```python
from build123d import *

# Parameters (mm, degrees)
SKETCH1_W           = 26
SKETCH1_H           = 26
BOSS_EXTRUDE1_DEPTH = 155
SHELL1_T            = -3
SKETCH2_W           = 10
SKETCH2_H           = 149
CUT_EXTRUDE1_DEPTH  = 3
SKETCH3_W           = 30
SKETCH3_H           = 26
BOSS_EXTRUDE2_DEPTH = 22
SKETCH4_R           = 2.2
CUT_EXTRUDE2_DEPTH  = 180.52715672


with BuildPart() as part:
    # Sketch1 → Boss-Extrude1 (new body)
    with BuildSketch(Plane(origin=(0, 0, 0), x_dir=(1, 0, 0), z_dir=(0, 1, 0))):
        Rectangle(SKETCH1_W, SKETCH1_H)
    extrude(amount=BOSS_EXTRUDE1_DEPTH)

    # Shell1
    shell1_openings = [part.faces().sort_by_distance(p)[0] for p in [
        (0, 155, 0),
        (0, 0, 0),
    ]]
    offset(amount=SHELL1_T, openings=shell1_openings, kind=Kind.INTERSECTION)

    # Sketch2 → Cut-Extrude1 (cut)
    with BuildSketch(Plane.XY.offset(13)):
        with Locations((0, 77.5)):
            Rectangle(SKETCH2_W, SKETCH2_H)
    extrude(amount=-CUT_EXTRUDE1_DEPTH, mode=Mode.SUBTRACT)

    # Sketch3 → Boss-Extrude2 (add)
    with BuildSketch(Plane(origin=(0, 155, 0), x_dir=(1, 0, 0), z_dir=(0, 1, 0))):
        Rectangle(SKETCH3_W, SKETCH3_H)
    extrude(amount=BOSS_EXTRUDE2_DEPTH)

    # Sketch4 → Cut-Extrude2 (cut, through all)
    with BuildSketch(Plane.XY.offset(13)):
        with Locations((0, 171)):
            Circle(SKETCH4_R)
    extrude(amount=-CUT_EXTRUDE2_DEPTH, mode=Mode.SUBTRACT)


solid = part.part
```
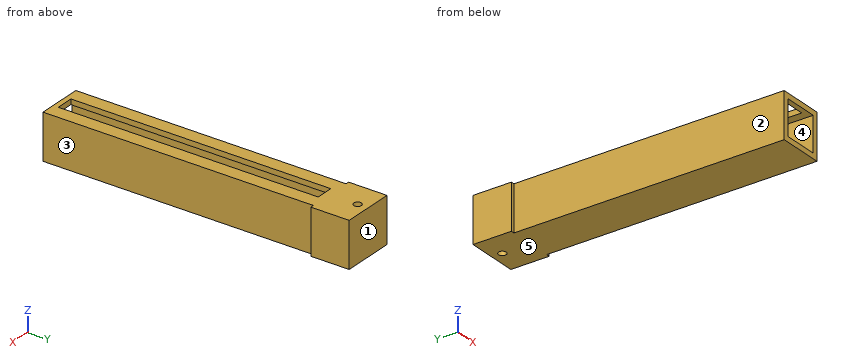
Read the model definition and answer for the solid it produces. Units are mm, in the model's axes. Face numbers are marked on the shaded views. A direction names the side the tool comes from. Round coordinates to 2 decimals unless told otherwise and drop trailing zeros. Write each loop counter-clockwise with the first axis right and the second up, starting at its lowest first coordinate (ties: lowest second). Pieces come first, ordered by that corner, then holes. Notation, with made-up numbers: (62.5, -9) -> (113.5, -9) arc R18 ccw to (113.5, -4) -> close; hole circle Ø1 at (26.25, -9.5). An arc over 180 degrees is marked (long way). Answer in a Markdown table with one row per item. Add a question column.
1) Consider line 1 (Y direction, x = 0, z = 4.5); line 2 (X direction, y = 9.5, z = -5.5); line 3 (Y direction, x = 0.75, z = 11.25). Determine where each line is inside the solid, lowest interval first.
2) Find section A-A, the plane x = 0. Determine the outline of the cut face in (y, z).
3) Given P1, Ø0.6, axis at x = -14, z = -2, coming from the -Y side; P2, Ø2.5, axis at y = 103, z = 12, coming from the +X side; P3, Ø6, axis at y = 106.5, z = 1.5, coming from the -X side, each flat-ended and moving along its own axis, determine where each tip first touches the part or whether it passes through.
4) Find section D-D, the plane y = 131. Determine the outline of the cut face in (x, z), and give its area (3 significant figures).
5) Find section B-B, the plane y = 171. Determine the outline of the cut face in (x, z), and give its area (3 significant figures).
6) Which of the six approach directions +Z, -Z, +X, -X, +Y, -Y give full straight-line access (tool end or side, diameter ignored) to the marked faces 1 and 2?
7) Determine the mould class of the marked faces 3, 4 and 5 for opening direction X: pulls with the +X half, pulls with the -X half, needs draft (parallel to the pull), parting line crosses it, or undercut.
8) Find section C-C, the plane x = -7.75. Determine the outline of the cut face in (y, z), and give its area (3 significant figures).
Findings below:
| question | item | result |
|---|---|---|
| 1 | line 1 | 155 to 168.8, 173.2 to 177 |
| 1 | line 2 | -13 to -10, 10 to 13 |
| 1 | line 3 | 0 to 3, 152 to 168.93, 173.07 to 177 |
| 2 | outline | (0, -13) -> (168.8, -13) -> (168.8, 13) -> (152, 13) -> (152, 10) -> (155, 10) -> (155, -10) -> (0, -10) -> close; (0, 10) -> (3, 10) -> (3, 13) -> (0, 13) -> close; (173.2, -13) -> (177, -13) -> (177, 13) -> (173.2, 13) -> close |
| 3 | P1 | y = 155 |
| 3 | P2 | x = 13 |
| 3 | P3 | x = -13 |
| 4 | outline | (-13, -13) -> (13, -13) -> (13, 13) -> (5, 13) -> (5, 10) -> (10, 10) -> (10, -10) -> (-10, -10) -> (-10, 10) -> (-5, 10) -> (-5, 13) -> (-13, 13) -> close |
| 4 | area | 246 mm² |
| 5 | outline | (-15, -13) -> (-2.2, -13) -> (-2.2, 13) -> (-15, 13) -> close; (2.2, -13) -> (15, -13) -> (15, 13) -> (2.2, 13) -> close |
| 5 | area | 666 mm² |
| 6 | face 1 | +Z, -Z, +X, -X, +Y |
| 6 | face 2 | +Z, -Z, -X, -Y |
| 7 | face 3 | pulls with the +X half |
| 7 | face 4 | undercut |
| 7 | face 5 | needs draft |
| 8 | outline | (0, -13) -> (177, -13) -> (177, 13) -> (0, 13) -> (0, 10) -> (155, 10) -> (155, -10) -> (0, -10) -> close |
| 8 | area | 1,500 mm² |
